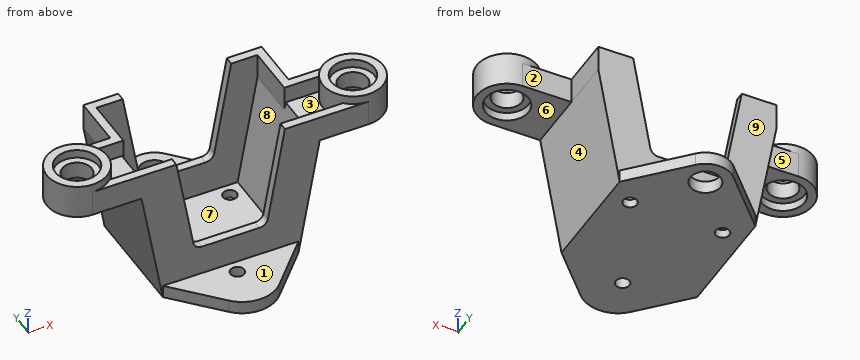
from build123d import *

# Parameters (mm, degrees)
ESTRUSIONE_ESTRUSIONE1_DEPTH = 3
SCHIZZO2_W                   = 20.66
SCHIZZO2_H                   = 13
ESTRUSIONE_ESTRUSIONE2_DEPTH = 14
TAGLIO_ESTRUSIONE1_DEPTH     = 25.91345219
SVUOTA1_T                    = -1
SCHIZZO4_R                   = 3.5
ESTRUSIONE_ESTRUSIONE3_DEPTH = 4
SCHIZZO5_R                   = 2.5
TAGLIO_ESTRUSIONE2_DEPTH     = 1
SCHIZZO6_R                   = 1.7
TAGLIO_ESTRUSIONE3_DEPTH     = 28.728326671
ESTRUSIONE_ESTRUSIONE4_DEPTH = 1.5
SCHIZZO8_R                   = 1.75
TAGLIO_ESTRUSIONE4_DEPTH     = 31.677517827
SCHIZZO9_R                   = 0.8
TAGLIO_ESTRUSIONE5_DEPTH     = 1.5
TAGLIO_ESTRUSIONE6_DEPTH     = 32.238759578
RACCORDO1_R                  = 1
SPECCHIA12_START             = 9
SPECCHIA12_DEPTH             = 1
RACCORDO2_R                  = 1
SPECCHIA15_START             = 9
SPECCHIA15_DEPTH             = 1
SCHIZZO12_R                  = 0.8
ESTRUSIONE_ESTRUSIONE5_DEPTH = 1.5
TAGLIO_ESTRUSIONE7_START     = -1
SCHIZZO13_R                  = 2.5
TAGLIO_ESTRUSIONE7_DEPTH     = 1


# Read off the part's stored shape, not the designer's step: Specchia12, Specchia15
with BuildPart() as part:
    # Schizzo1 → Estrusione-Estrusione1 (new body)
    with BuildSketch(Plane.XY):
        Polygon((-15.99, 4), (-10.33, 4), (-10.33, 10), (10.33, 10), (10.33, 4), (15.99, 4), (15.99, -3), (-15.99, -3), align=None)
    extrude(amount=ESTRUSIONE_ESTRUSIONE1_DEPTH)

    # Schizzo2 → Estrusione-Estrusione2 (add)
    with BuildSketch(Plane.XY):
        with Locations((0, 3.5)):
            Rectangle(SCHIZZO2_W, SCHIZZO2_H)
    extrude(amount=-ESTRUSIONE_ESTRUSIONE2_DEPTH)

    # Schizzo3 → Taglio-Estrusione1 (cut, through all)
    with BuildSketch(Plane(origin=(0, 10, 0), x_dir=(1, 0, 0), z_dir=(0, 1, 0))):
        Polygon((-10.33, 0), (-7.86142227, 14), (-10.33, 14), align=None)
    taglio_estrusione1 = extrude(amount=-TAGLIO_ESTRUSIONE1_DEPTH, mode=Mode.SUBTRACT)

    # Specchia1: Taglio-Estrusione1 across plane
    add(taglio_estrusione1.mirror(Plane(origin=(0, 0, 0), x_dir=(0, 0, 1), z_dir=(1, 0, 0))), mode=Mode.SUBTRACT)

    # Svuota1
    svuota1_openings = [part.faces().sort_by_distance(p)[0] for p in [
        (0, 2.81654304, 3),
    ]]
    offset(amount=SVUOTA1_T, openings=svuota1_openings, kind=Kind.INTERSECTION)

    # Schizzo4 → Estrusione-Estrusione3 (add)
    with BuildSketch(Plane.XY):
        with Locations(Location((-15.99, 0.5, 0), (0, 0, 270))):
            Circle(SCHIZZO4_R)
    estrusione_estrusione3 = extrude(amount=ESTRUSIONE_ESTRUSIONE3_DEPTH)

    # Schizzo5 → Taglio-Estrusione2 (cut)
    with BuildSketch(Plane.XY.offset(4)):
        with Locations((-15.99, 0.5)):
            Circle(SCHIZZO5_R)
    taglio_estrusione2 = extrude(amount=-TAGLIO_ESTRUSIONE2_DEPTH, mode=Mode.SUBTRACT)

    # Schizzo6 → Taglio-Estrusione3 (cut, through all)
    with BuildSketch(Plane.XY.offset(3)):
        with Locations((-15.99, 0.5)):
            Circle(SCHIZZO6_R)
    taglio_estrusione3 = extrude(amount=-TAGLIO_ESTRUSIONE3_DEPTH, mode=Mode.SUBTRACT)

    # Specchia2: Estrusione-Estrusione3, Taglio-Estrusione2, Taglio-Estrusione3 across plane
    add(estrusione_estrusione3.mirror(Plane(origin=(0, 0, 0), x_dir=(0, 0, 1), z_dir=(1, 0, 0))))
    add(taglio_estrusione2.mirror(Plane(origin=(0, 0, 0), x_dir=(0, 0, 1), z_dir=(1, 0, 0))), mode=Mode.SUBTRACT)
    add(taglio_estrusione3.mirror(Plane(origin=(0, 0, 0), x_dir=(0, 0, 1), z_dir=(1, 0, 0))), mode=Mode.SUBTRACT)

    # Schizzo7 → Estrusione-Estrusione4 (add)
    with BuildSketch(Plane(origin=(0, 0, -14), x_dir=(-1, 0, 0), z_dir=(0, 0, -1))):
        with BuildLine():
            Line((-7.86142227, 10), (-2.188751242, 16.051674439))
            ThreePointArc((-2.188751242, 16.051674439), (0, 17), (2.188751242, 16.051674439))
            Line((2.188751242, 16.051674439), (7.86142227, 10))
            Line((7.86142227, 10), (-7.86142227, 10))
        make_face()
    extrude(amount=-ESTRUSIONE_ESTRUSIONE4_DEPTH)

    # Schizzo8 → Taglio-Estrusione4 (cut, through all)
    with BuildSketch(Plane.XY.offset(-12.5)):
        with Locations((0, 14)):
            Circle(SCHIZZO8_R)
    extrude(amount=-TAGLIO_ESTRUSIONE4_DEPTH, mode=Mode.SUBTRACT)

    # Schizzo9 → Taglio-Estrusione5 (cut)
    with BuildSketch(Plane(origin=(0, 0, -14), x_dir=(-1, 0, 0), z_dir=(0, 0, -1))):
        with Locations((-5.36142227, 7.5)):
            Circle(SCHIZZO9_R)
    taglio_estrusione5 = extrude(amount=-TAGLIO_ESTRUSIONE5_DEPTH, mode=Mode.SUBTRACT)

    # Specchia5: Taglio-Estrusione5 across plane
    add(taglio_estrusione5.mirror(Plane(origin=(0, 0, 0), x_dir=(0, 0, 1), z_dir=(1, 0, 0))), mode=Mode.SUBTRACT)

    # Schizzo10 → Taglio-Estrusione6 (cut, through all)
    with BuildSketch(Plane.XZ.offset(3)):
        Polygon((-6.289561189, 3), (-4.17363742, -9), (4.17363742, -9), (6.289561189, 3), align=None)
    extrude(amount=-TAGLIO_ESTRUSIONE6_DEPTH, mode=Mode.SUBTRACT)

    # Raccordo1
    raccordo1_edges = [part.edges().sort_by_distance(p)[0] for p in [
        (-4.17363742, -2.5, -9),
    ]]
    fillet(raccordo1_edges, radius=RACCORDO1_R)

    # Specchia12 outline → Specchia12 (add)
    with BuildSketch(Plane(origin=(0, 0, 0), x_dir=(1, 0, 0), z_dir=(0, 1, 0)).offset(SPECCHIA12_START)):
        with BuildLine():
            ThreePointArc((-4.319345542, 8.173648178), (-3.977325399, 8.766044443), (-3.334537789, 9))
            Line((-3.334537789, 9), (-4.17363742, 9))
            Line((-4.17363742, 9), (-4.319345542, 8.173648178))
        make_face()
    extrude(amount=SPECCHIA12_DEPTH)

    # Raccordo2
    raccordo2_edges = [part.edges().sort_by_distance(p)[0] for p in [
        (4.17363742, -2.5, -9),
    ]]
    fillet(raccordo2_edges, radius=RACCORDO2_R)

    # Specchia15 outline → Specchia15 (add)
    with BuildSketch(Plane(origin=(0, 0, 0), x_dir=(1, 0, 0), z_dir=(0, 1, 0)).offset(SPECCHIA15_START)):
        with BuildLine():
            ThreePointArc((3.334537789, 9), (3.977325399, 8.766044443), (4.319345542, 8.173648178))
            Line((4.319345542, 8.173648178), (4.17363742, 9))
            Line((4.17363742, 9), (3.334537789, 9))
        make_face()
    extrude(amount=SPECCHIA15_DEPTH)

    # Schizzo12 → Estrusione-Estrusione5 (add)
    with BuildSketch(Plane(origin=(0, 0, -14), x_dir=(-1, 0, 0), z_dir=(0, 0, -1))):
        with BuildLine():
            Line((-7.86142227, -3), (-2.918334989, -8.273345625))
            ThreePointArc((-2.918334989, -8.273345625), (0, -9.537779706), (2.918334989, -8.273345625))
            Line((2.918334989, -8.273345625), (7.86142227, -3))
            Line((7.86142227, -3), (-7.86142227, -3))
        make_face()
        with Locations((0, -4.5)):
            Circle(SCHIZZO12_R, mode=Mode.SUBTRACT)
    extrude(amount=-ESTRUSIONE_ESTRUSIONE5_DEPTH)

    # Schizzo13 → Taglio-Estrusione7 (cut)
    with BuildSketch(Plane(origin=(0, 0, 0), x_dir=(-1, 0, 0), z_dir=(0, 0, -1)).offset(TAGLIO_ESTRUSIONE7_START)):
        with Locations((-15.99, 0.5)):
            Circle(SCHIZZO13_R)
    taglio_estrusione7 = extrude(amount=TAGLIO_ESTRUSIONE7_DEPTH, mode=Mode.SUBTRACT)

    # Specchia16: Taglio-Estrusione7 across plane
    add(taglio_estrusione7.mirror(Plane(origin=(0, 0, 0), x_dir=(0, 0, 1), z_dir=(1, 0, 0))), mode=Mode.SUBTRACT)


solid = part.part
Design review of the part built by this model. Coordinates are the model's own, in mm. Face numbers are marked on the shaded views. A direction names the side the tool comes from. Round coordinates to 2 decimals unless told otherwise and drop trailing zeros. Write each loop counter-clockwise with the first axis right and the second up, starting at its lowest first coordinate (ties: lowest second). Pieces come first, ordered by that corner, then holes.
Item 1: Consider section D-D on z = -7.25. Give the boundary of the cut face in (x, y).
Item 2: Consider section B-B on z = 1.5. Give the boundary of the cut face in (x, y).
Item 3: Consider section A-A on x = 0. Give the boundary of the cut face in (y, z).
Item 4: For pin 1 Ø5 at (x, z) = (-2, -2) entering from -Y; pin 2 Ø3 at (x, y) = (-11.5, 0.5) entering from +Z; pin 3 Ø3 at (x, z) = (5.5, -2) entering from -Y; pin 4 Ø2.5 at (x, z) = (12.5, 1) entering from +Y, all flat-tipped, find the tip position at first contact; note any pin that passes through.
Item 5: Draft analysis for pull direction Y (two halves, no side actions). For the marked faces 6, 7, 8 and 9, state which applies: released by +Y, released by -Y, zero draft, split by the parting line, or undercut.
Item 6: Wall thickness on L1, parallel to Y at x = 0, z = -13.35; L2, parallel to X at y = 6.5, z = 2; L3, parallel to Y at x = -15.99, z = 0.35: over which ranges is each line inside the solid? List them lowest first.
Item 7: For the marked faces 1, 2, 3, 4 and 5, list the 3-axis set-ups (+Z, -Z, +X, -X, +Y, -Y) from which the entire face can be reached by the end or side of a thin tool; tool diameter is ignored.
Item 8: Consider section C-C on y = -4.5. Give the boundary of the cut face in (x, z).
Check values:
1. outline: (-9.05, -3) - (-4.48, -3) - (-4.48, -2) - (-8.04, -2) - (-8.04, 9) - (-4.48, 9) - (-4.48, 10) - (-9.05, 10) - close; (4.48, -3) - (9.05, -3) - (9.05, 10) - (4.48, 10) - (4.48, 9) - (8.04, 9) - (8.04, -2) - (4.48, -2) - close
2. outline: (-15.99, -3) - (-6.03, -3) - (-6.03, -2) - (-13.54, -2) arc R3.5 ccw to (-13.54, 3) - (-9.33, 3) - (-9.33, 9) - (-6.03, 9) - (-6.03, 10) - (-10.33, 10) - (-10.33, 4) - (-15.99, 4) arc R3.5 ccw to start; (6.03, -3) - (15.99, -3) arc R3.5 ccw to (15.99, 4) - (10.33, 4) - (10.33, 10) - (6.03, 10) - (6.03, 9) - (9.33, 9) - (9.33, 3) - (13.54, 3) arc R3.5 ccw to (13.54, -2) - (6.03, -2) - close; hole circle Ø3.4 at (-15.99, 0.5); hole circle Ø3.4 at (15.99, 0.5)
3. outline: (-9.54, -14) - (-5.3, -14) - (-5.3, -12.5) - (-9.54, -12.5) - close; (-3.7, -14) - (12.25, -14) - (12.25, -12.5) - (10, -12.5) - (10, -9) - (9, -9) - (9, -13) - (-2, -13) - (-2, -9) - (-3, -9) - (-3, -12.5) - (-3.7, -12.5) - close; (15.75, -14) - (17, -14) - (17, -12.5) - (15.75, -12.5) - close
4. pin 1: passes through
4. pin 2: stops at z = 4
4. pin 3: stops at y = -3
4. pin 4: stops at y = 4
5. face 6: zero draft
5. face 7: undercut
5. face 8: undercut
5. face 9: released by +Y
6. L1: y = -9.54 to -5.3, -3.7 to 12.25, 15.75 to 17
6. L2: x = -10.33 to -9.33, 9.33 to 10.33
6. L3: y = -3 to -2, 3 to 4
7. face 1: +Z, +X, -X, -Y
7. face 2: +Z, -Z, +X, +Y
7. face 3: +Z
7. face 4: -Z, +X, +Y, -Y
7. face 5: +Z, -Z, -X, +Y
8. outline: (-6.46, -14) - (-0.8, -14) - (-0.8, -12.5) - (-6.46, -12.5) - close; (0.8, -14) - (6.46, -14) - (6.46, -12.5) - (0.8, -12.5) - close
